Part model, mm, in its own coordinate system. Round coordinates to 2 decimals unless told otherwise and drop trailing zeros. Write each loop counter-clockwise with the first axis right and the second up, starting at its lowest first coordinate (ties: lowest second). Pieces come first, ordered by that corner, then holes.
1) Drill centre lines: L1, parallel to Y at x = 128, z = 4.25; L2, parallel to Y at x = 190.5, z = 5; L3, parallel to X at y = -420, z = 4.5. Where is each one in solid material? Low to high.
2) Saw through at B-B on y = -49.5. Write the cut outline in (x, z).
3) Saw through at A-A on z = 2.5. Write the cut outline in (x, y), and give its area (3 significant figures).
4) Saw through at C-C on x = 209.5. Write the cut outline in (y, z), and give its area (3 significant figures).
5) Flat gauge pins, fed straight in: pin 1 (3 mm diameter, centred on x = 256, z = 4.5, fed in from +Y); pin 2 (1 mm diameter, centred on x = 100, y = -169.5, fed in from -Z); pin 3 (2 mm diameter, centred on y = -354, z = 4.5, fed in from +X); pin 4 (3 mm diameter, centred on y = -55.5, z = 1.5, fed in from +X). Where does each tip first touch, or does it go through?
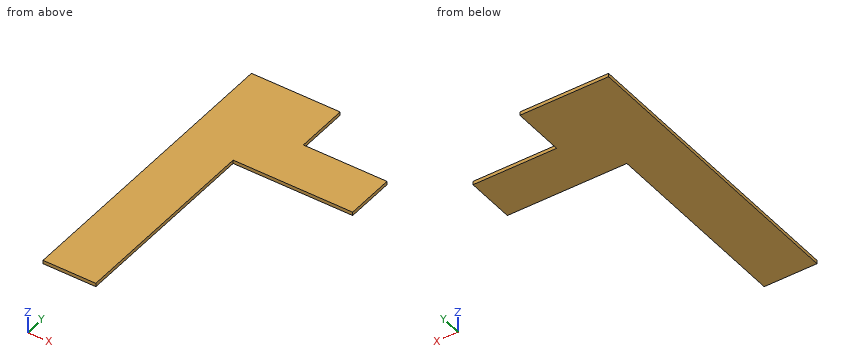
Autodesk Inventor part; units mm, degrees
ref_plane "YZ Plane" through (0, 0, 0) normal (1, 0, 0) x (0, 1, 0)
ref_plane "XZ Plane" through (0, 0, 0) normal (0, 1, 0) x (-1, 0, 0)
ref_plane "XY Plane" through (0, 0, 0) normal (0, 0, 1) x (1, 0, 0)
sketch "Sketch1" plane through (0, 0, 0) normal (0, 0, 1) x (1, 0, 0)
  line L0 (0, 0) -> (307.2255, 0)
  line L1 (307.2255, 0) -> (307.2255, -177.8)
  line L2 (307.2255, -177.8) -> (0, -177.8)
  line L3 (0, -177.8) -> (0, 0)
  line L4 (460.8382, 266.0651) -> (307.2255, 0)
  line L5 (307.2255, 0) -> (0, 0)
  line L6 (0, 0) -> (-153.6127, 266.0651)
  line L7 (-153.6127, 266.0651) -> (0, 532.1302)
  line L8 (0, 532.1302) -> (307.2255, 532.1302)
  line L9 (307.2255, 532.1302) -> (460.8382, 266.0651)
  point P0 (153.6127, 266.0651)
  dimension "d1" = 177.8
  dimension "d39" = 307.2255
extrude "Extrusion1" add sketch "Sketch1" along normal blind 6.35 contours L0 L1 L2 L3
sketch "Sketch2" plane through (0, 0, 0) normal (0, 1, 0) x (1, 0, 0)
  line L0 (307.2255, -6.35) -> (0, -6.35)
  line L1 (0, -6.35) -> (-3.6662, -6.35)
  line L2 (-3.6662, -6.35) -> (0, 0)
  line L3 (0, 0) -> (0, -6.35)
  line L4 (0, 0) -> (0, -6.35)
  line L5 (0, -6.35) -> (0, 0)
  line L6 (307.2255, -6.35) -> (310.8917, -6.35)
  line L7 (307.2255, 0) -> (307.2255, -6.35)
  line L8 (310.8917, -6.35) -> (307.2255, 0)
  line L9 (307.2255, 0) -> (307.2255, -6.35)
  dimension "d4" = 30
  dimension "d5" = 60
extrude "Extrusion2" add sketch "Sketch2" against normal blind 177.8
sketch "Sketch3" plane through (0, 0, 6.35) normal (0, 0, 1) x (1, 0, 0)
  line L0 (81.3338, -88.9) -> (281.3338, -88.9)
  line L1 (281.3338, -88.9) -> (281.3338, 0)
  line L2 (281.3338, 0) -> (81.3338, 0)
  line L3 (81.3338, 0) -> (81.3338, -88.9)
  line L4 (-3.6662, 0) -> (310.8917, 0)
  line L5 (81.3338, -88.9) -> (192.81, -88.9)
  line L6 (121.05, 0) -> (81.3338, 0)
  line L7 (81.3338, 0) -> (81.3338, -88.9)
  line L8 (281.3338, 0) -> (169.304, 0)
  line L9 (156.3338, -88.9) -> (281.3338, -88.9)
  line L10 (281.3338, -88.9) -> (281.3338, 0)
  line L11 (81.3338, 0) -> (156.3338, 0)
  line L12 (156.3338, 0) -> (156.3338, -88.9)
  line L13 (156.3338, -88.9) -> (81.3338, -88.9)
  line L14 (81.3338, -88.9) -> (81.3338, 0)
  line L15 (281.3338, 0) -> (281.3338, -88.9)
  line L16 (281.3338, -88.9) -> (281.3338, 0)
  line L17 (-3.6662, 0) -> (-3.6662, -177.8)
  point P0 (0, 0)
  point P1 (281.3338, -44.45)
  point P2 (153.6127, 0)
  point P3 (153.6127, 0)
  dimension "d8" = 200
  dimension "d9" = 88.9
  dimension "d14" = 75
  dimension "d33" = 85
extrude "Extrusion3" cut sketch "Sketch3" against normal through all contours L12 L2 L1 L0
sketch "Sketch5" plane through (0, 0, 6.35) normal (0, 0, 1) x (1, 0, 0)
  line L0 (310.8917, -177.8) -> (-3.6662, -177.8)
  line L1 (-3.6662, -177.8) -> (91.5838, -177.8)
  line L2 (91.5838, -177.8) -> (91.5838, -533.4)
  line L3 (91.5838, -533.4) -> (-3.6662, -533.4)
  line L4 (-3.6662, -533.4) -> (-3.6662, -177.8)
  point P0 (0, 0)
  dimension "d23" = 95.25
  dimension "d24" = 355.6
extrude "Extrusion5" add sketch "Sketch5" against normal blind 10
sketch "Sketch6" plane through (-3.6662, -177.8, -3.65) normal (0, 1, 0) x (1, 0, 0)
  line L0 (0, -10) -> (3.6662, -3.65)
  line L1 (0, 0) -> (95.25, 0)
  line L2 (0, -10) -> (0, 0)
  line L3 (95.25, -3.65) -> (3.6662, -3.65)
  line L4 (95.25, -3.65) -> (95.25, 0)
  point P0 (3.6662, -3.65)
extrude "Extrusion6" cut sketch "Sketch6" against normal through all
sketch "Sketch9" plane through (0, 0, 6.35) normal (0, 0, 1) x (1, 0, 0)
  line L0 (281.3338, -88.9) -> (156.3338, -88.9)
  line L1 (310.8917, 0) -> (310.8917, -177.8)
  line L2 (281.3338, -88.9) -> (310.8917, -88.9)
  line L3 (310.8917, -88.9) -> (310.8917, 0)
  line L4 (310.8917, 0) -> (281.3338, 0)
  line L5 (281.3338, 0) -> (281.3338, -88.9)
  point P0 (0, 0)
extrude "Extrusion8" cut sketch "Sketch9" against normal through all
sketch "Sketch10" plane through (0, 0, 0) normal (0, 1, 0) x (1, 0, 0)
  line L0 (0, 0) -> (0, -6.35)
  line L1 (-3.6662, -6.35) -> (156.3338, -6.35)
  line L2 (0, -6.35) -> (-3.6662, -6.35)
  line L3 (0, 0) -> (-3.6662, -6.35)
  line L4 (0, 0) -> (-3.6662, -6.35)
  line L5 (0, 0) -> (156.3338, 0)
  line L6 (-3.6662, -6.35) -> (0, 0)
  line L7 (156.3338, 0) -> (307.2255, 0)
  line L8 (307.2255, 0) -> (307.2255, -6.35)
  line L9 (310.8917, -6.35) -> (156.3338, -6.35)
  line L10 (307.2255, -6.35) -> (310.8917, -6.35)
  line L11 (307.2255, 0) -> (310.8917, -6.35)
  line L12 (310.8917, -6.35) -> (307.2255, 0)
  line L13 (307.2255, 0) -> (310.8917, -6.35)
extrude "Extrusion9" cut sketch "Sketch10" against normal through all contours L0 L1 L3 | L11 L9 L8
sketch "Sketch11" plane through (0, 0, 6.35) normal (0, 0, 1) x (1, 0, 0)
  line L0 (0, 0) -> (-3.6662, 0)
  line L1 (-3.6662, 0) -> (-3.6662, -533.4)
  line L2 (-3.6662, -533.4) -> (0, -533.4)
  line L3 (0, -533.4) -> (0, 0)
  line L4 (91.5838, -177.8) -> (91.5838, -533.4)
  dimension "d40" = 95.25
extrude "Extrusion10" add sketch "Sketch11" against normal blind 6.35
sketch "Sketch12" plane through (0, 0, 6.35) normal (0, 0, 1) x (1, 0, 0)
  line L0 (-3.6662, 0) -> (156.3338, 0)
  line L1 (156.3338, 0) -> (-3.6662, 0)
  line L2 (-3.6662, 0) -> (-3.6662, 6.35)
  line L3 (-3.6662, 6.35) -> (156.3338, 6.35)
  line L4 (156.3338, 6.35) -> (156.3338, 0)
  point P0 (0, 0)
  point P1 (-3.6662, 3.175)
  dimension "d43" = 6.35
extrude "Extrusion11" add sketch "Sketch12" against normal blind 6.35
properties part number "BA03" material "ABS Plastic"
Completed:
1. L1: y = -177.8 to 6.35
1. L2: y = -177.8 to -88.9
1. L3: x = -3.67 to 91.58
2. outline: (-3.67, 0) - (156.33, 0) - (156.33, 6.35) - (-3.67, 6.35) - close
3. outline: (-3.67, -533.4) - (91.58, -533.4) - (91.58, -177.8) - (307.23, -177.8) - (307.23, -88.9) - (156.33, -88.9) - (156.33, 6.35) - (-3.67, 6.35) - close
3. area: 76,700 mm2
4. outline: (-177.8, 0) - (-88.9, 0) - (-88.9, 6.35) - (-177.8, 6.35) - close
4. area: 565 mm2
5. pin 1: stops at y = -88.9
5. pin 2: stops at z = 0
5. pin 3: stops at x = 91.58
5. pin 4: stops at x = 156.33
